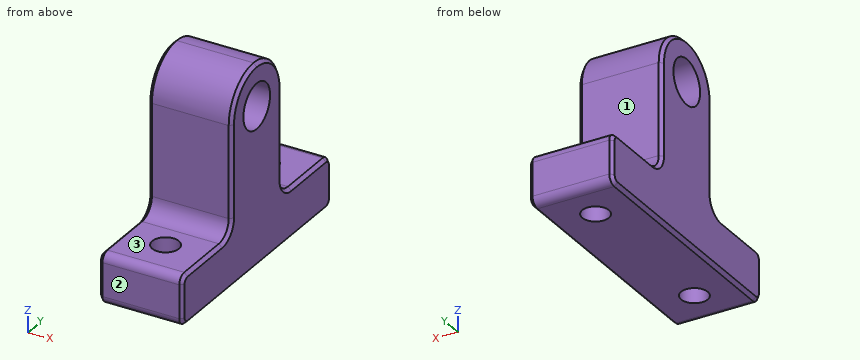
Autodesk Inventor part; units mm, degrees
ref_plane "Plano de trabajo1" through (-7.3035, 18.7537, -25.5454) normal (-1, 0, 0) x (0, 1, 0)
ref_plane "YZ Plane" through (0, 0, 0) normal (1, 0, 0) x (0, 1, 0)
ref_plane "XZ Plane" through (0, 0, 0) normal (0, 1, 0) x (-1, 0, 0)
ref_plane "Plano de trabajo1" through (-7.3035, 18.7537, -25.5454) normal (-1, 0, 0) x (0, 1, 0)
sketch "Boceto1" plane through (-7.3035, 18.7537, -25.5454) normal (-1, 0, 0) x (0, 1, 0)
  line L0 (40.0076, 19) -> (-60.0081, 19) construction
  line L1 (15, 19) -> (-15, 19)
  line L2 (-15, 19) -> (-15, 13)
  line L3 (-15, 13) -> (15, 13)
  line L4 (15, 13) -> (15, 19)
  line L5 (-5, 19) -> (5, 19)
  line L6 (5, 19) -> (5, -5)
  line L7 (5, -5) -> (-5, -5)
  line L8 (-5, -5) -> (-5, 19)
  arc A0 (-1.0724, -0.9) -> (-0.9, -1.0724) centre (0, 0) ccw construction
  circle A1 centre (0, 0) radius 2.7
  point P0 (-18.7537, -25.5454)
  point P1 (0, 19)
  point P2 (0, -5)
  point P3 (-5, 13)
  point P4 (5, 13)
  dimension "d0" = 6
  dimension "d1" = 30
  dimension "d2" = 5.4
  dimension "d3" = 0
  dimension "d4" = 0
  dimension "d5" = 10
  dimension "d6" = 5
extrude "Extrusión1" add sketch "Boceto1" against normal blind 10
sketch "Boceto2" plane through (-7.3035, 23.7537, -38.5454) normal (0, 0, 1) x (1, 0, 0)
  line L0 (0, 0) -> (10, 0) construction
  line L1 (0, 0) -> (0, 10) construction
  line L2 (0, -20) -> (0, -10) construction
  line L3 (0, -10) -> (10, -10) construction
  point P0 (7.3035, -23.7537)
  point P1 (5, 5)
  point P2 (5, -15)
  point P3 (5, 0)
  point P4 (5, -10)
  dimension "d9" = 5
  dimension "d10" = 5
  dimension "d11" = 5
  dimension "d12" = 5
hole "Agujero1" at (-2.3035, 28.7537, -38.5454) at (-2.3035, 8.7537, -38.5454) direction (0, 0, -1) diameter 3.2 end through all
fillet "Empalme1" radius 5 2 edges at (-2.3035, 23.7537, -20.5454) (-2.3035, 13.7537, -20.5454)
fillet "Empalme2" radius 1 4 edges at (-2.3035, 33.7537, -38.5454) (-2.3035, 3.7537, -38.5454) (-2.3035, 33.7537, -44.5454) (-2.3035, 3.7537, -44.5454)
fillet "Empalme3" radius 2 2 edges at (-2.3035, 23.7537, -38.5454) (-2.3035, 13.7537, -38.5454)
chamfer "Chaflán1" distance 0.4 angle 45 24 edges at (-7.3035, 29.2537, -38.5454) (-7.3035, 33.4608, -38.8383) (-7.3035, 33.7537, -41.5454) (-7.3035, 33.4608, -44.2525) (-7.3035, 18.7537, -44.5454) (-7.3035, 4.0466, -44.2525) (-7.3035, 3.7537, -41.5454) (-7.3035, 4.0466, -38.8383) (-7.3035, 8.2537, -38.5454) (-7.3035, 13.7537, -31.0451) (-7.3035, 22.2894, -22.0097) (-7.3035, 23.7537, -31.0451) (2.6965, 29.2537, -38.5454) (2.6965, 23.7537, -31.0451) (2.6965, 22.2894, -22.0097) (2.6965, 13.7537, -31.0451) (2.6965, 8.2537, -38.5454) (2.6965, 4.0466, -38.8383) (2.6965, 3.7537, -41.5454) (2.6965, 4.0466, -44.2525) (2.6965, 18.7537, -44.5454) (2.6965, 33.4608, -44.2525) (2.6965, 33.7537, -41.5454) (2.6965, 33.4608, -38.8383)
properties part number "SoporteEjeMotor"
For this review, take the finished solid that the model builds, in its own axes (mm). Face numbers are marked on the shaded views. A direction names the side the tool comes from. Round coordinates to 2 decimals unless told otherwise and drop trailing zeros. Order: outer loops, then holes, each group sorted by start corner. A loop starts at its lowest first (then second) coordinate and runs counter-clockwise, first axis right, second up.
Q1. Wall thickness on line 1 (Y direction, x = -1.5, z = -41.5); line 2 (Z direction, x = -4.25, y = 30); line 3 (Y direction, x = -0.5, z = -36): over which ranges is each line inside the solid? List them lowest first.
Findings below:
line 1: y = 3.75 to 7.37, 10.14 to 27.37, 30.14 to 33.75
line 2: z = -44.55 to -38.55
line 3: y = 13.75 to 23.75
Q2. We need section D-D, the plane z = -41. Give the boundary of the cut face in (x, y).
Findings below:
outline: (-7.3, 4.15) - (-6.9, 3.75) - (2.3, 3.75) - (2.7, 4.15) - (2.7, 33.35) - (2.3, 33.75) - (-6.9, 33.75) - (-7.3, 33.35) - close; hole circle Ø3.2 at (-2.3, 8.75); hole circle Ø3.2 at (-2.3, 28.75)
Q3. Machinability: for the marked faces 1, 2 and 3, which of the approach directions +Z, -Z, +X, -X, +Y, -Y give a long, thin tool a straight path to every point of the face, cutting with its end or side? Answer none if there is none.
Findings below:
face 1: +Z, +X, -X, +Y
face 2: +Z, -Z, +X, -X, -Y
face 3: +Z, +X, -X, -Y
Q4. We need section A-A, the plane y = 28. Give the boundary of the cut face in (x, z).
Findings below:
outline: (-7.3, -44.15) - (-6.9, -44.55) - (-3.71, -44.55) - (-3.71, -38.55) - (-6.9, -38.55) - (-7.3, -38.95) - close; (-0.89, -44.55) - (2.3, -44.55) - (2.7, -44.15) - (2.7, -38.95) - (2.3, -38.55) - (-0.89, -38.55) - close
Q5. Insertion check: P1, Ø2.5, axis at x = -2.3, y = 8.75, coming from the -Z side; P2, Ø1.5, axis at x = 0.5, z = -33.5, coming from the -Y side; P3, Ø5.5, axis at x = -1, y = 30, coming from the +Z side. Each pin has a flat end and moves straight along its axis. Give the tip position at first contact, or say it passes through.
Findings below:
P1: passes through
P2: stops at y = 13.75
P3: stops at z = -38.55
Q6. We need section B-B, the plane x = -1.75. State how many separate pieces and enclosed holes the cut face has, plus the area to 3 significant figures.
Findings below:
separate pieces: 3
enclosed holes: 1
area: 291 mm2
Q7. We need section C-C, the plane z = -27.25. Give the boundary of the cut face in (x, y), plus the area to 3 significant figures.
Findings below:
outline: (-7.3, 14.15) - (-6.9, 13.75) - (2.3, 13.75) - (2.7, 14.15) - (2.7, 16.66) - (-7.3, 16.66) - close; (-7.3, 20.85) - (2.7, 20.85) - (2.7, 23.35) - (2.3, 23.75) - (-6.9, 23.75) - (-7.3, 23.35) - close
area: 57.8 mm2
